Part model, mm, in its own coordinate system. A direction names the side the tool comes from. Round coordinates to 2 decimals unless told otherwise and drop trailing zeros. Loops run counter-clockwise (first coordinate to the right, second up) from the corner with the lowest first, then second, coordinate; pieces in that order, holes last. Notation, with made-up numbers: (-32.75, 87.5) - (-18.75, 87.5) arc R14 ccw to (-18.75, 93.5) - close; hole circle Ø6 at (50, 44.5). An arc over 180 degrees is marked (long way). Put each result on its own line as item: value.
from build123d import *

# Parameters (mm, degrees)
F1_DEPTH = 63.5
F2_DEPTH = 25.4
F3_DEPTH = 15.875
F5_R     = 6.35


with BuildPart() as f1:
    # F0 (on Front) → F1 (new body, symmetric)
    with BuildSketch(Plane.XZ):
        Polygon((-41.275, 9.525), (-41.275, -9.525), (41.275, -9.525), (41.275, 9.525), (22.225, 9.525), align=None)
    extrude(amount=F1_DEPTH, both=True)

    # F0 (on Front) → F2 (join, symmetric)
    with BuildSketch(Plane.XZ):
        with BuildLine():
            Line((22.225, 9.525), (41.275, 9.525))
            Line((41.275, 9.525), (41.275, 27.0002))
            ThreePointArc((41.275, 27.0002), (45.9246798487, 38.2255201513), (57.15, 42.8752))
            Line((57.15, 42.8752), (60.325, 42.8752))
            Line((60.325, 42.8752), (60.325, 61.9252))
            Line((60.325, 61.9252), (57.15, 61.9252))
            add(Edge.make_bspline(
                [(54.201505188, 61.8005161386), (55.2055384053, 61.8594589572), (56.1890341086, 61.9011525736), (57.15, 61.9252)],
                knots=[108.3967265897, 108.3967265897, 108.3967265897, 108.3967265897, 111.5045361635, 111.5045361635, 111.5045361635, 111.5045361635], degree=3))
            ThreePointArc((54.201505188, 61.8005161386), (31.4329647285, 50.6304713028), (22.225, 27.0002))
            Line((22.225, 27.0002), (22.225, 9.525))
        make_face()
        Polygon((85.8293095101, 61.9252), (60.325, 61.9252), (60.325, 42.8752), (85.7459063837, 42.8752), align=None)
    extrude(amount=F2_DEPTH, both=True)

    # F0 (on Front) → F3 (join)
    with BuildSketch(Plane.XZ):
        with BuildLine():
            add(Edge.make_bspline(
                [(-41.275, 9.525), (-40.8220224818, 36.7045980931), (19.1820126646, 59.7446602565), (54.201505188, 61.8005161386)],
                knots=[0, 0, 0, 0, 108.3967265897, 108.3967265897, 108.3967265897, 108.3967265897], degree=3))
            Line((-41.275, 9.525), (22.225, 9.525))
            Line((22.225, 9.525), (22.225, 27.0002))
            ThreePointArc((22.225, 27.0002), (31.4329647285, 50.6304713028), (54.201505188, 61.8005161386))
        make_face()
    extrude(amount=F3_DEPTH)

    # F0 (on Front) → F4 (revolve)
    with BuildSketch(Plane.XZ):
        Polygon((85.8501046896, 66.675), (85.8293095101, 61.9252), (85.7459063837, 42.8752), (85.725, 38.1), (111.125, 38.1), (111.125, 66.675), align=None)
    revolve(axis=Axis((85.7875523448, 0, 52.3875), (0.0043780749, 0, 0.9999904162)))

    # F5
    f5_edges = [f1.edges().sort_by_distance(p)[0] for p in [
        (41.275, -63.5, 0),
        (-41.275, -63.5, 0),
        (41.275, 63.5, 0),
        (-41.275, 63.5, 0),
    ]]
    fillet(f5_edges, radius=F5_R)


solid = f1.part
1. Tool access for faces 1 (the flat face through (41.275, -1, 4)), 2 (the flat face through (22.225, 13, 18)), 3 (the flat face through (47, 25.4, 42)): list every direction of +Z, -Z, +X, -X, +Y, -Y with a clear straight run to the whole face (end or side of a thin tool).
A:
face 1: -Z, +X, +Y, -Y
face 2: +Z, -X, +Y
face 3: +Z, +X, -X, +Y
2. Two-plate mould, pull along X, no slides. Class faces 4 (the flat face through (60, 0, 42.875)), 5 (the flat face through (1, 31, 9.525)), 6 (the flat face through (-41.275, -1, 0)): pulls with the +X half, pulls with the -X half, needs draft (parallel to the pull), parting line crosses it, or undercut.
A:
face 4: undercut
face 5: needs draft
face 6: pulls with the -X half
3. Band-saw the part on A-A (y = 31.5). List the corners of the cut face in (x, z) (3 decimals), plus the area to 3 significant figures.
A:
outline: (-41.275, -9.525) - (41.275, -9.525) - (41.275, 9.525) - (-41.275, 9.525) - close
area: 1,570 mm²
4. Probe line 1 along Y through (x, z) = (36.5, 44.5); line 2 along X through (y, z) = (-30.5, 6) (3 decimals); line 3 along Y through (x, z) = (-33, 20) (3 decimals). List the from-to ranges inside material, lowest first. Write a range as [from, to].
A:
line 1: y = [-25.4, 25.4]
line 2: x = [-41.275, 41.275]
line 3: y = [-15.875, 0]
5. Pin check, flat tips, straight feed: P1, Ø2, axis at x = -8, y = -16, coming from the +Z side; P2, Ø7.5, axis at y = -18.5, z = 16.5, coming from the -X side; P3, Ø3, axis at x = 55.5, y = 21.5, coming from the +Z side. Stop position of each tip, or through.
A:
P1: stops at z = 44.84
P2: stops at x = -40.71
P3: stops at z = 61.92
